Design review of the part built by this model. Coordinates are the model's own, in mm. Face numbers are marked on the shaded views. Coordinates: 2 decimals unless noted, no trailing zeros. Loops run counter-clockwise (first coordinate to the right, second up) from the corner with the lowest first, then second, coordinate; pieces in that order, holes last. Notation, with made-up numbers: (24, 89) -> (66, 89) arc R21 cw to (66, 106) -> close; hole circle Ø8 at (28.25, 6.5). An arc over 180 degrees is marked (long way). One line per item, written item: value. Start each with the question number.
1. Insertion check: pin 1 (6 mm diameter, centred on y = 61, z = -4, fed in from +X) (3 decimals); pin 2 (3 mm diameter, centred on y = 93.5, z = -4.5, fed in from -X); pin 3 (1.5 mm diameter, centred on x = 15, y = 44.5, fed in from -Z); pin 4 (18 mm diameter, centred on x = 0, z = 0, fed in from +Y). Each pin has a flat end and moves straight along its axis. Give the tip position at first contact, or say it passes through.
2. Add section A-A on z = 0. Write out the cut boundary in (x, y).
3. Add section C-C on y = 64. Write out the cut boundary in (x, z), plus the area to 3 significant figures.
4. Add section B-B on x = 0. Write out the cut boundary in (y, z), plus the area to 3 significant figures.
5. For probe 1 along X at (y, z) = (69, 0); probe 2 along Y at (x, z) = (14, 0), list the stretches that pass through material, from the lowest coordinate up.
6. Draft analysis for pull direction Z (two halves, no side actions). For the marked faces 1, 2 and 3, state which applies: pulls with the +Z half, pulls with the -Z half, needs draft (parallel to the pull), parting line crosses it, or undercut.
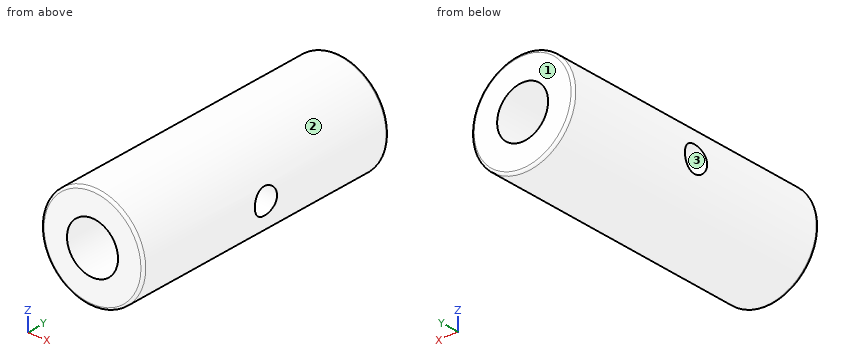
```python
from build123d import *

# Parameters (mm, degrees)
SKETCH_1_R               = 20
SKETCH_1_R_2             = 10
EXTRUDE_1_DEPTH          = 110
SKETCH_2_R               = 5
CUT_EXTRUDE_1_DEPTH      = 21
CUT_EXTRUDE_1_DEPTH_BACK = 21
FILLET_1_R               = 1


with BuildPart() as part:
    # 草图1 → 凸台-拉伸1 (new body)
    with BuildSketch(Plane(origin=(0, 0, 0), x_dir=(1, 0, 0), z_dir=(0, 1, 0))):
        Circle(SKETCH_1_R)
        Circle(SKETCH_1_R_2, mode=Mode.SUBTRACT)
    extrude(amount=EXTRUDE_1_DEPTH)

    # 草图2 → 切除-拉伸1 (cut, two sides)
    with BuildSketch(Plane(origin=(0, 0, 0), x_dir=(0, 0, -1), z_dir=(1, 0, 0))) as cut_extrude_1_sk:
        with Locations((0, 55)):
            Circle(SKETCH_2_R)
    extrude(amount=CUT_EXTRUDE_1_DEPTH, mode=Mode.SUBTRACT)
    extrude(cut_extrude_1_sk.sketch, amount=-CUT_EXTRUDE_1_DEPTH_BACK, mode=Mode.SUBTRACT)

    # 圆角1
    fillet_1_edges = [part.edges().sort_by_distance(p)[0] for p in [
        (-20, 0, 0),
        (-20, 110, 0),
    ]]
    fillet(fillet_1_edges, radius=FILLET_1_R)


solid = part.part
```
Worked answers:
1. pin 1: stops at x = 19.975
1. pin 2: stops at x = -19.77
1. pin 3: stops at z = -14.03
1. pin 4: passes through
2. outline: (-20, 1) arc R1 ccw to (-19, 0) -> (-10, 0) -> (-10, 50) -> (-20, 50) -> close; (-20, 60) -> (-10, 60) -> (-10, 110) -> (-19, 110) arc R1 ccw to (-20, 109) -> close; (10, 0) -> (19, 0) arc R1 ccw to (20, 1) -> (20, 50) -> (10, 50) -> close; (10, 60) -> (20, 60) -> (20, 109) arc R1 ccw to (19, 110) -> (10, 110) -> close
3. outline: circle Ø40 at (0, 0); hole circle Ø20 at (0, 0)
3. area: 942 mm²
4. outline: (0, -19) arc R1 ccw to (1, -20) -> (109, -20) arc R1 ccw to (110, -19) -> (110, -10) -> (0, -10) -> close; (0, 10) -> (110, 10) -> (110, 19) arc R1 ccw to (109, 20) -> (1, 20) arc R1 ccw to (0, 19) -> close
4. area: 2,200 mm²
5. probe 1: x = -20 to -10, 10 to 20
5. probe 2: y = 0 to 50, 60 to 110
6. face 1: needs draft
6. face 2: parting line crosses it
6. face 3: undercut
